Geometry check sheet. Reference: drawing and pictorial views, mm from the part's lowest x, y, z. Coordinates: 2 decimals unless noted, no trailing zeros. Loops run counter-clockwise (first coordinate to the right, second up) from the corner with the lowest first, then second, coordinate; pieces in that order, holes last.
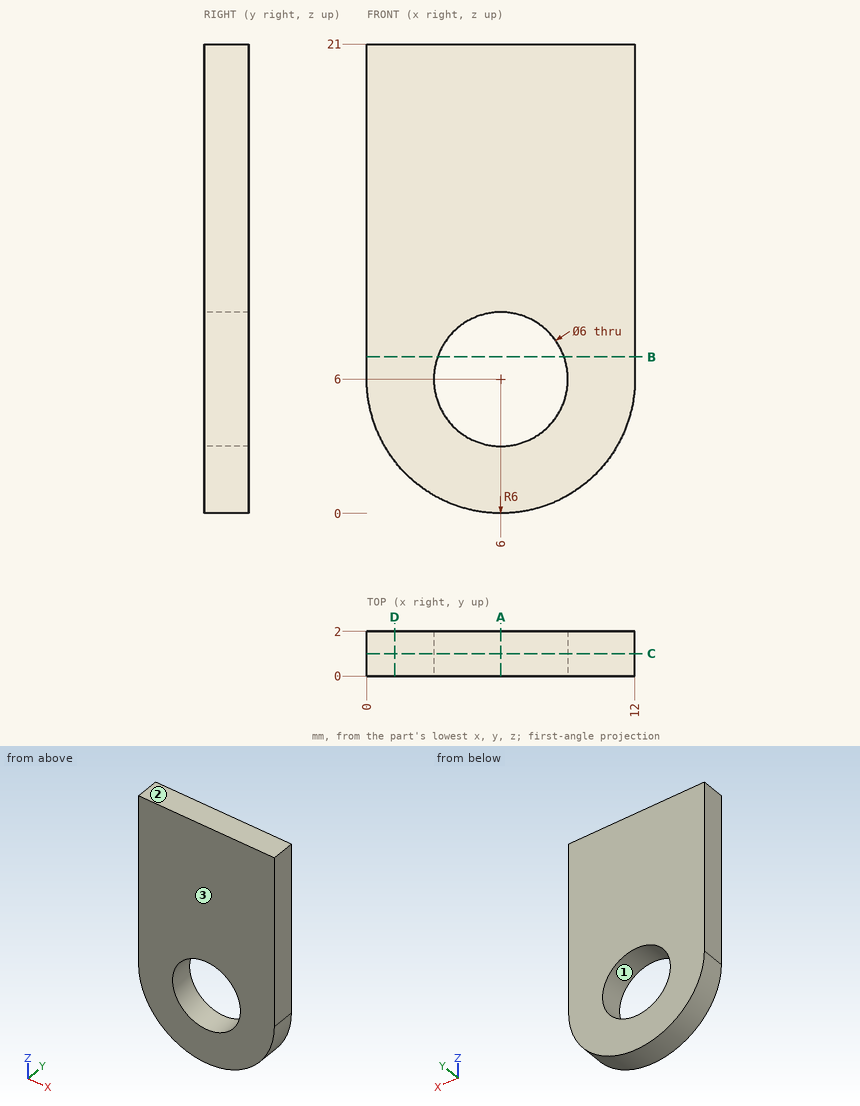
1) Mould release check, pull along Z, two halves, no side actions. Record for the marked faces 1, 2 and 3: +Z half, -Z half, draft (parallel to the pull), parting line (faces both ways), or undercut.
Data:
face 1: undercut
face 2: +Z half
face 3: draft
2) Section check B-B on z = 7. Record the cut outline in (x, y).
Data:
outline: (0, 0) - (3.17, 0) - (3.17, 2) - (0, 2) - close; (8.83, 0) - (12, 0) - (12, 2) - (8.83, 2) - close
3) Material ranges on probe 1 along Z at (x, y) = (6, 0.85); probe 2 along Z at (x, y) = (4.25, 0.6); probe 3 along X at (y, z) = (1.3, 6.75), recorded low to high.
Data:
probe 1: z = 0 to 3, 9 to 21
probe 2: z = 0.26 to 3.56, 8.44 to 21
probe 3: x = 0 to 3.1, 8.9 to 12
4) Section check A-A on x = 6. Record the cut outline in (y, z).
Data:
outline: (0, 0) - (2, 0) - (2, 3) - (0, 3) - close; (0, 9) - (2, 9) - (2, 21) - (0, 21) - close
5) Section check C-C on y = 1. Record the cut outline in (x, z), and give its area (3 significant figures).
Data:
outline: (0, 6) arc R6 ccw to (12, 6) - (12, 21) - (0, 21) - close; hole circle Ø6 at (6, 6)
area: 208 mm2
6) Section check D-D on x = 1.25. Record the cut outline in (y, z).
Data:
outline: (0, 2.33) - (2, 2.33) - (2, 21) - (0, 21) - close
